The model under review builds one solid part; all positions refer to its coordinate system, in mm. A direction names the side the tool comes from. Coordinates: 2 decimals unless noted, no trailing zeros. Order: outer loops, then holes, each group sorted by start corner. A loop starts at its lowest first (then second) coordinate and runs counter-clockwise, first axis right, second up. Notation, with made-up numbers: M 35.5,60.25 L 56.5,60.25 A18 ccw 56.5,75.25 Z; hole C 25,-17 d7. An arc over 180 degrees is marked long. One line per item, written item: value.
```python
from build123d import *

# Parameters (mm, degrees)
SKETCH_1_R      = 1
EXTRUDE_1_DEPTH = 2.5
SKETCH_1_3_R    = 3.5
SKETCH_1_3_R_2  = 1.5
EXTRUDE_2_DEPTH = 4.8


with BuildPart() as part:
    # Sketch 1 → Extrude 1 (new body)
    with BuildSketch(Plane(origin=(0, 0, 0), x_dir=(1, 0, 0), z_dir=(0, 1, 0))):
        with BuildLine():
            ThreePointArc((-0.305925926, -3.486604269), (-3.5, 0), (-0.305925926, 3.486604269))
            Line((-0.305925926, 3.486604269), (-13.702785185, 2.311120544))
            ThreePointArc((-13.702785185, 2.311120544), (-15.82, 0), (-13.702785185, -2.311120544))
            Line((-13.702785185, -2.311120544), (-0.305925926, -3.486604269))
        make_face()
        with Locations((-13.5, 0)):
            Circle(SKETCH_1_R, mode=Mode.SUBTRACT)
        with Locations((-11, 0)):
            Circle(SKETCH_1_R, mode=Mode.SUBTRACT)
        with Locations((-8.5, 0)):
            Circle(SKETCH_1_R, mode=Mode.SUBTRACT)
        with Locations((-6, 0)):
            Circle(SKETCH_1_R, mode=Mode.SUBTRACT)
    extrude(amount=EXTRUDE_1_DEPTH)

    # Sketch 1_3 → Extrude 2 (add)
    with BuildSketch(Plane(origin=(0, 0, 0), x_dir=(1, 0, 0), z_dir=(0, 1, 0))):
        Circle(SKETCH_1_3_R)
        Circle(SKETCH_1_3_R_2, mode=Mode.SUBTRACT)
    extrude(amount=EXTRUDE_2_DEPTH)


solid = part.part
```
(1) We need section C-C, the plane x = 1.25. State the section outline as (y, z) points.
Geometry results:
outline: M 0,-3.27 L 4.8,-3.27 L 4.8,-0.83 L 0,-0.83 Z; M 0,0.83 L 4.8,0.83 L 4.8,3.27 L 0,3.27 Z
(2) For L1, parallel to X at y = 1.45, z = 0; L2, parallel to X at y = 3, z = 0; L3, parallel to X at y = 1.2, z = 0.5, list the stretches that pass through material, from the lowest coordinate up.
Geometry results:
L1: x = -15.82 to -14.5, -12.5 to -12, -10 to -9.5, -7.5 to -7, -5 to -1.5, 1.5 to 3.5
L2: x = -3.5 to -1.5, 1.5 to 3.5
L3: x = -15.77 to -14.37, -12.63 to -11.87, -10.13 to -9.37, -7.63 to -6.87, -5.13 to -1.41, 1.41 to 3.46
(3) We need section A-A, the plane y = 0.9. State the section outline as (x, z) points.
Geometry results:
outline: M -13.7,-2.31 L -0.31,-3.49 A3.5 ccw long -0.31,3.49 L -13.7,2.31 A2.32 ccw Z; hole C -13.5,0 d2; hole C -11,0 d2; hole C -8.5,0 d2; hole C -6,0 d2; hole C 0,0 d3
(4) Tool access review of faces 4 (the cylindrical face through (-9.3, 1.2, 0.6)), 5 (the cylindrical face through (3.233, 2.9, 1.341)): name each direction out of +Z, -Z, +X, -X, +Y, -Y from which nothing blocks a thin tool from reaching the whole face with its end or side.
Geometry results:
face 4: +Y, -Y
face 5: +Y
(5) We need section B-B, the plane z = 0. State the section outline as (x, y) points.
Geometry results:
outline: M -15.82,0 L -14.5,0 L -14.5,2.5 L -15.82,2.5 Z; M -12.5,0 L -12,0 L -12,2.5 L -12.5,2.5 Z; M -10,0 L -9.5,0 L -9.5,2.5 L -10,2.5 Z; M -7.5,0 L -7,0 L -7,2.5 L -7.5,2.5 Z; M -5,0 L -1.5,0 L -1.5,4.8 L -3.5,4.8 L -3.5,2.5 L -5,2.5 Z; M 1.5,0 L 3.5,0 L 3.5,4.8 L 1.5,4.8 Z
(6) Insertion check: pin 1 Ø1.5 at (y, z) = (1.5, 1.5) entering from -X; pin 2 Ø2.5 at (x, z) = (-13.5, 0) entering from +Y; pin 3 Ø2 at (x, z) = (-7, -0.5) entering from -Y. Each pin has a flat end and moves straight along its axis. Give the tip position at first contact, or say it passes through.
Geometry results:
pin 1: stops at x = -15.7
pin 2: stops at y = 2.5
pin 3: stops at y = 0
(7) We need section D-D, the plane z = -1.25. State the section outline as (x, y) points, plus the area to 3 significant figures.
Geometry results:
outline: M -15.45,0 L -0.83,0 L -0.83,4.8 L -3.27,4.8 L -3.27,2.5 L -15.45,2.5 Z; M 0.83,0 L 3.27,0 L 3.27,4.8 L 0.83,4.8 Z
area: 53.9 mm2
(8) Mouldability with a two-part tool opening along X and no side actions: class faces 1 (the cylindrical face through (-12.546, 1.232, -0.3)), 2 (the flat face through (-6.911, 1.232, -2.907)), 3 (the flat face through (0, 4.8, 2)) as +X half, -X half, draft (parallel to the pull), parting line (faces both ways), or undercut.
Geometry results:
face 1: undercut
face 2: -X half
face 3: draft
